Read the model definition and answer for the solid it produces. Units are mm, in the model's axes. Give positions to 0.01 mm unless a question says otherwise; leave off trailing zeros. Order: outer loops, then holes, each group sorted by start corner. A loop starts at its lowest first (then second) coordinate and runs counter-clockwise, first axis right, second up. Notation, with made-up numbers: (-3, -32) -> (46, -32) arc R20 cw to (46, -5) -> close; hole circle Ø8 at (44, 5.5). An arc over 180 degrees is marked (long way). Use one line per item in the form item = value.
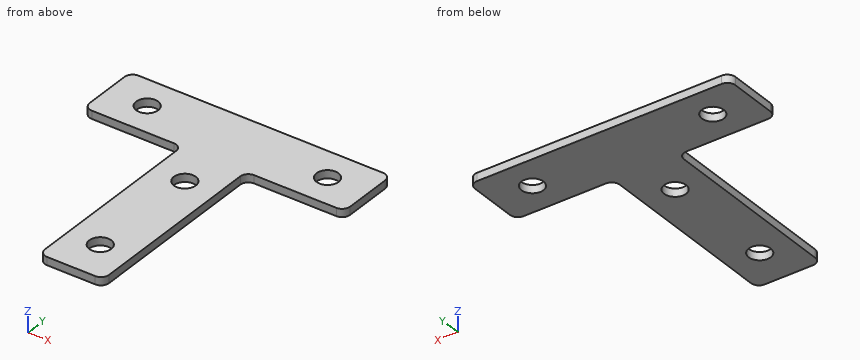
Autodesk Inventor part; units mm, degrees
ref_plane "YZ Plane" through (0, 0, 0) normal (1, 0, 0) x (0, 1, 0)
ref_plane "XZ Plane" through (0, 0, 0) normal (0, 1, 0) x (-1, 0, 0)
ref_plane "XY Plane" through (0, 0, 0) normal (0, 0, 1) x (1, 0, 0)
sketch "草图1" plane through (0, 0, 0) normal (0, 0, 1) x (1, 0, 0)
  line L0 (32.5, -8) -> (-32.5, -8)
  line L1 (-32.5, -8) -> (-32.5, 8)
  line L2 (-32.5, 8) -> (32.5, 8)
  line L3 (32.5, 8) -> (32.5, -8)
  line L4 (32.5, -8) -> (-32.5, 8) construction
  line L5 (-32.5, -8) -> (32.5, 8) construction
  line L6 (8, -57) -> (-8, -57)
  line L7 (-8, -57) -> (-8, 8)
  line L8 (-8, 8) -> (8, 8)
  line L9 (8, 8) -> (8, -57)
  line L10 (8, -57) -> (-8, 8) construction
  line L11 (-8, -57) -> (8, 8) construction
  line L12 (0, 0) -> (0, -24.5)
  point P0 (-8, -8)
  point P1 (8, -8)
  dimension "d0" = 65
  dimension "d1" = 16
  dimension "d2" = 49
  dimension "d3" = 16
extrude "拉伸1" add sketch "草图1" along normal blind 2
sketch "草图2" plane through (0, 0, 2) normal (0, 0, 1) x (1, 0, 0)
  line L0 (-32.5, 8) -> (-32.5, -8)
  line L1 (-32.5, 0) -> (32.5, 0)
  line L2 (32.5, -8) -> (32.5, 8)
  line L3 (0, 8) -> (0, -57)
  line L4 (-8, -57) -> (8, -57)
  circle A0 centre (-22.5, 0) radius 2.75
  circle A1 centre (0, -18) radius 2.75
  circle A2 centre (0, -47) radius 2.75
  circle A3 centre (22.5, 0) radius 2.75
  point P0 (0, 0)
  dimension "d6" = 22.5
  dimension "d7" = 5.5
  dimension "d8" = 5.5
  dimension "d9" = 5.5
  dimension "d10" = 29
  dimension "d11" = 10
extrude "拉伸2" cut sketch "草图2" against normal blind 10
fillet "圆角1" radius 2 8 edges at (-8, -8, 1) (-32.5, -8, 1) (-32.5, 8, 1) (32.5, -8, 1) (-8, -57, 1) (8, -57, 1) (8, -8, 1) (32.5, 8, 1)
equation "\"d12\" = d11"
properties part number "T型"
Item 1: The part is cut by section D-D on z = 0.95. Give the vertices of the cut face in (x, y), and give its area (3 significant figures).
Checks:
outline = (-32.5, -6) arc R2 ccw to (-30.5, -8) -> (-10, -8) arc R2 cw to (-8, -10) -> (-8, -55) arc R2 ccw to (-6, -57) -> (6, -57) arc R2 ccw to (8, -55) -> (8, -10) arc R2 cw to (10, -8) -> (30.5, -8) arc R2 ccw to (32.5, -6) -> (32.5, 6) arc R2 ccw to (30.5, 8) -> (-30.5, 8) arc R2 ccw to (-32.5, 6) -> close; hole circle Ø5.5 at (-22.5, 0); hole circle Ø5.5 at (0, -47); hole circle Ø5.5 at (0, -18); hole circle Ø5.5 at (22.5, 0)
area = 1,730 mm²
Item 2: The part is cut by section A-A on y = -18. Give the vertices of the cut face in (x, z).
Checks:
outline = (-8, 0) -> (-2.75, 0) -> (-2.75, 2) -> (-8, 2) -> close; (2.75, 0) -> (8, 0) -> (8, 2) -> (2.75, 2) -> close
Item 3: Given pin 1 Ø0.6 at (x, z) = (18, 1) entering from -Y; pin 2 Ø3.5 at (x, y) = (0, -47) entering from -Z; pin 3 Ø0.6 at (y, z) = (-41, 0.5) entering from +X, each flat-ended and moving along its own axis, determine where each tip first touches the part or whether it passes through.
Checks:
pin_1 = -8
pin_2 = through
pin_3 = 8
Item 4: Straight lines are drawn through the part: L1, parallel to X at y = 0, z = 1.2; L2, parallel to Y at x = 0, z = 1.2; L3, parallel to X at y = -18, z = 0.4. For each, find the intervals that lie inside material, in ascending order. Write a range as from..to.
Checks:
L1 = -32.5..-25.25, -19.75..19.75, 25.25..32.5
L2 = -57..-49.75, -44.25..-20.75, -15.25..8
L3 = -8..-2.75, 2.75..8
Item 5: The part is cut by section C-C on y = 0. Give the vertices of the cut face in (x, z), and give its area (3 significant figures).
Checks:
outline = (-32.5, 0) -> (-25.25, 0) -> (-25.25, 2) -> (-32.5, 2) -> close; (-19.75, 0) -> (19.75, 0) -> (19.75, 2) -> (-19.75, 2) -> close; (25.25, 0) -> (32.5, 0) -> (32.5, 2) -> (25.25, 2) -> close
area = 108 mm²
